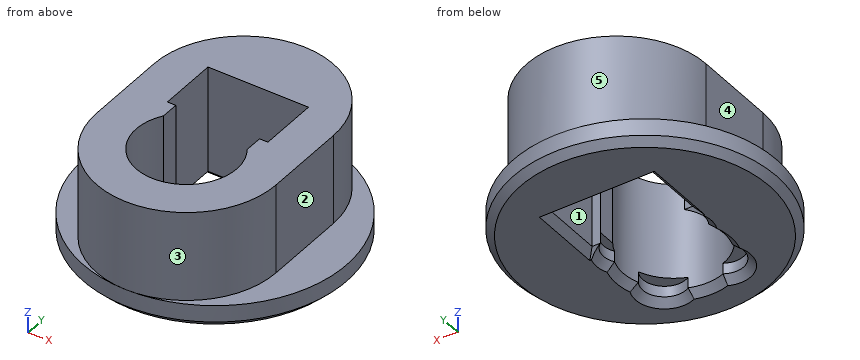
```python
from build123d import *

# Parameters (mm, degrees)
EXTRUDE_1_DEPTH        = 9.5
SKETCH_8_R             = 11
EXTRUDE_2_DEPTH        = 2
CUT_EXTRUDE_1105_DEPTH = 21.530465168
CUT_EXTRUDE_1724_DEPTH = 1.5
CHAMFER_1_SIZE         = 0.6


with BuildPart() as part:
    # Эскиз7 → Бобышка-Вытянуть1 (new body)
    with BuildSketch(Plane.XY):
        with BuildLine():
            Line((-7.5, 0), (-7.5, 7))
            ThreePointArc((-7.5, 7), (0, 14.5), (7.5, 7))
            Line((7.5, 7), (7.5, 0))
            ThreePointArc((7.5, 0), (0, -7.5), (-7.5, 0))
        make_face()
    extrude(amount=EXTRUDE_1_DEPTH)

    # Эскиз8 → Бобышка-Вытянуть2 (add)
    with BuildSketch(Plane(origin=(0, 0, 0), x_dir=(-1, 0, 0), z_dir=(0, 0, -1))):
        with Locations((0, 3.5)):
            Circle(SKETCH_8_R)
    extrude(amount=-EXTRUDE_2_DEPTH)

    # Эскиз3 → Cut-Extrude 1105 (cut, through all)
    with BuildSketch(Plane(origin=(0, 0, 0), x_dir=(-1, 0, 0), z_dir=(0, 0, -1))):
        with BuildLine():
            Line((-4.2, 8.8), (4.2, 8.8))
            Line((4.2, 8.8), (4.2, 3.821637353))
            Line((4.2, 3.821637353), (3.5, 3.821637353))
            Line((3.5, 3.821637353), (3.5, 2.321637353))
            ThreePointArc((3.5, 2.321637353), (0, -4.2), (-3.5, 2.321637353))
            Line((-3.5, 2.321637353), (-3.5, 3.821637353))
            Line((-3.5, 3.821637353), (-4.2, 3.821637353))
            Line((-4.2, 3.821637353), (-4.2, 8.8))
        make_face()
    extrude(amount=-CUT_EXTRUDE_1105_DEPTH, mode=Mode.SUBTRACT)

    # Эскиз6 → Cut-Extrude 1724 (cut)
    with BuildSketch(Plane(origin=(0, 0, 0), x_dir=(-1, 0, 0), z_dir=(0, 0, -1))):
        with BuildLine():
            ThreePointArc((-1.462331642, 3.937205376), (-3.676955262, 3.676955262), (-3.937205376, 1.462331642))
            ThreePointArc((-3.937205376, 1.462331642), (-2.969848481, 2.969848481), (-1.462331642, 3.937205376))
        make_face()
        with BuildLine():
            ThreePointArc((3.937205376, -1.462331642), (3.676955262, -3.676955262), (1.462331642, -3.937205376))
            ThreePointArc((1.462331642, -3.937205376), (2.969848481, -2.969848481), (3.937205376, -1.462331642))
        make_face()
        with BuildLine():
            ThreePointArc((-1.462331642, -3.937205376), (-2.969848481, -2.969848481), (-3.937205376, -1.462331642))
            ThreePointArc((-3.937205376, -1.462331642), (-3.676955262, -3.676955262), (-1.462331642, -3.937205376))
        make_face()
        with BuildLine():
            ThreePointArc((1.462331642, 3.937205376), (2.969848481, 2.969848481), (3.937205376, 1.462331642))
            ThreePointArc((3.937205376, 1.462331642), (3.676955262, 3.676955262), (1.462331642, 3.937205376))
        make_face()
    extrude(amount=-CUT_EXTRUDE_1724_DEPTH, mode=Mode.SUBTRACT)

    # Фаска1
    chamfer_1_edges = [part.edges().sort_by_distance(p)[0] for p in [
        (11, 3.5, 0),
        (4.2, 6.310818677, 0),
        (3.856775231, 3.821637353, 0),
        (-4.2, 6.310818677, 0),
        (0, 8.8, 0),
        (4.2, 0, 0),
        (0, -4.2, 0),
        (-4.2, 0, 0),
        (-3.856775231, 3.821637353, 0),
        (-4.175552206, 2.722821223, 0),
        (3.676955262, -3.676955262, 0),
        (-3.676955262, -3.676955262, 0),
        (4.175552206, 2.722821223, 0),
    ]]
    chamfer(chamfer_1_edges, length=CHAMFER_1_SIZE)


solid = part.part
```
Check sheet for the modelled part. Datum: model origin and axes. Units: mm. Face numbers are marked on the shaded views. A direction names the side the tool comes from. Round coordinates to 2 decimals unless told otherwise and drop trailing zeros. Loops run counter-clockwise (first coordinate to the right, second up) from the corner with the lowest first, then second, coordinate; pieces in that order, holes last. Notation, with made-up numbers: (-13, -4) - (44, -4) arc R36 cw to (44, 32) - close; hole circle Ø5 at (-2.75, 70.5). An arc over 180 degrees is marked (long way). Write item = value, one per line. Start each with the question number.
Q1. Section check A-A (z = 4.25). Record the boundary of the cut face in (x, y).
Q2. Thickness scan on L1, parallel to Y at x = 0, z = 4; L2, parallel to X at y = 0, z = 6; L3, parallel to Z at x = -7, y = -4. Record the ranges inside material, lowest first.
Q3. Depth check by flat-ended pin: P1, Ø1.4, axis at x = 2.5, y = -3, coming from the -Z side; P2, Ø0.8, axis at y = 3, z = 4.5, coming from the -X side; P3, Ø1, axis at x = -8, z = 2, coming from the -Y side. Enter the tip coordinate at first touch or a pass-through.
Q4. Access from +Z, -Z, +X, -X, +Y, -Y to the whole of each face (thin tool, end or side, straight path). Record for the marked faces 1, 2, 3, 4 and 5.
Derived:
q1.outline = (-7.5, 0) arc R7.5 ccw to (7.5, 0) - (7.5, 7) arc R7.5 ccw to (-7.5, 7) - close; hole (-4.2, 3.82) - (-3.5, 3.82) - (-3.5, 2.32) arc R4.2 ccw (long way) to (3.5, 2.32) - (3.5, 3.82) - (4.2, 3.82) - (4.2, 8.8) - (-4.2, 8.8) - close
q2.L1 = -7.5 to -4.2, 8.8 to 14.5
q2.L2 = -7.5 to -4.2, 4.2 to 7.5
q2.L3 = 0 to 2
q3.P1 = 1.5
q3.P2 = -7.5
q3.P3 = -4.55
q4.face_1 = +Z, -Z
q4.face_2 = +Z, +X, +Y, -Y
q4.face_3 = +Z, -Y
q4.face_4 = +Z, -X, +Y, -Y
q4.face_5 = +Z, +Y
